Design review of the part shown in the three views and the two pictorial views. Dimensions are in mm from the part's minimum x, y and z. Coordinates: 2 decimals unless noted, no trailing zeros. Order: outer loops, then holes, each group sorted by start corner. A loop starts at its lowest first (then second) coordinate and runs counter-clockwise, first axis right, second up. Notation, with made-up numbers: (79.25, 49) -> (114.25, 49) arc R30 ccw to (114.25, 78) -> close; hole circle Ø4 at (12, 77). An arc over 180 degrees is marked (long way). Answer as a JSON object with one key per item and string values. Group by question number.
1) Add section A-A, the plane y = 40.5. Write out the cut boundary in (x, z).
2) For pin 1 (1 mm diameter, centred on x = 17, y = 83.5, fed in from -Z); pin 2 (3 mm diameter, centred on x = 14.5, y = 86, fed in from +Z), all flat-tipped, find the tip position at first contact; note any pin that passes through.
3) Add section B-B, the plane x = 5.5. Write out the cut boundary in (y, z).
4) Add section C-C, the plane z = 0.3. Count the separate pieces of the cut face and the enclosed holes in it, then the cut area to 3 significant figures.
5) Wall thickness on L1, parallel to X at y = 33, z = 0.75: over which ranges is the line inside the solid? List them lowest first.
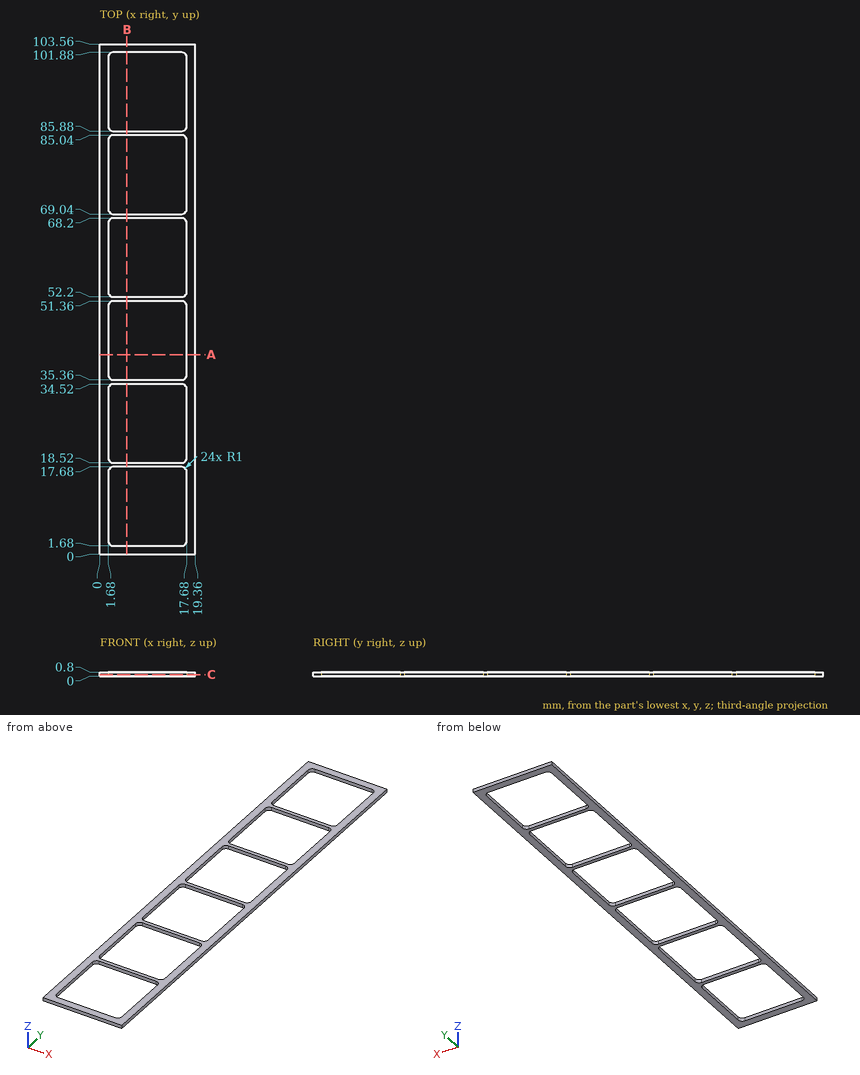
Output values:
{
 "1": {"outline": "(0, 0) -> (1.68, 0) -> (1.68, 0.8) -> (0, 0.8) -> close; (17.68, 0) -> (19.36, 0) -> (19.36, 0.8) -> (17.68, 0.8) -> close"},
 "2": {"pin 1": "passes through", "pin 2": "stops at z = 0.8"},
 "3": {"outline": "(0, 0) -> (1.68, 0) -> (1.68, 0.8) -> (0, 0.8) -> close; (17.68, 0) -> (18.52, 0) -> (18.52, 0.8) -> (17.68, 0.8) -> close; (34.52, 0) -> (35.36, 0) -> (35.36, 0.8) -> (34.52, 0.8) -> close; (51.36, 0) -> (52.2, 0) -> (52.2, 0.8) -> (51.36, 0.8) -> close; (68.2, 0) -> (69.04, 0) -> (69.04, 0.8) -> (68.2, 0.8) -> close; (85.04, 0) -> (85.88, 0) -> (85.88, 0.8) -> (85.04, 0.8) -> close; (101.88, 0) -> (103.56, 0) -> (103.56, 0.8) -> (101.88, 0.8) -> close"},
 "4": {"separate pieces": "1", "enclosed holes": "6", "area": "474 mm²"},
 "5": {"L1": "x = 0 to 1.68, 17.68 to 19.36"}
}
